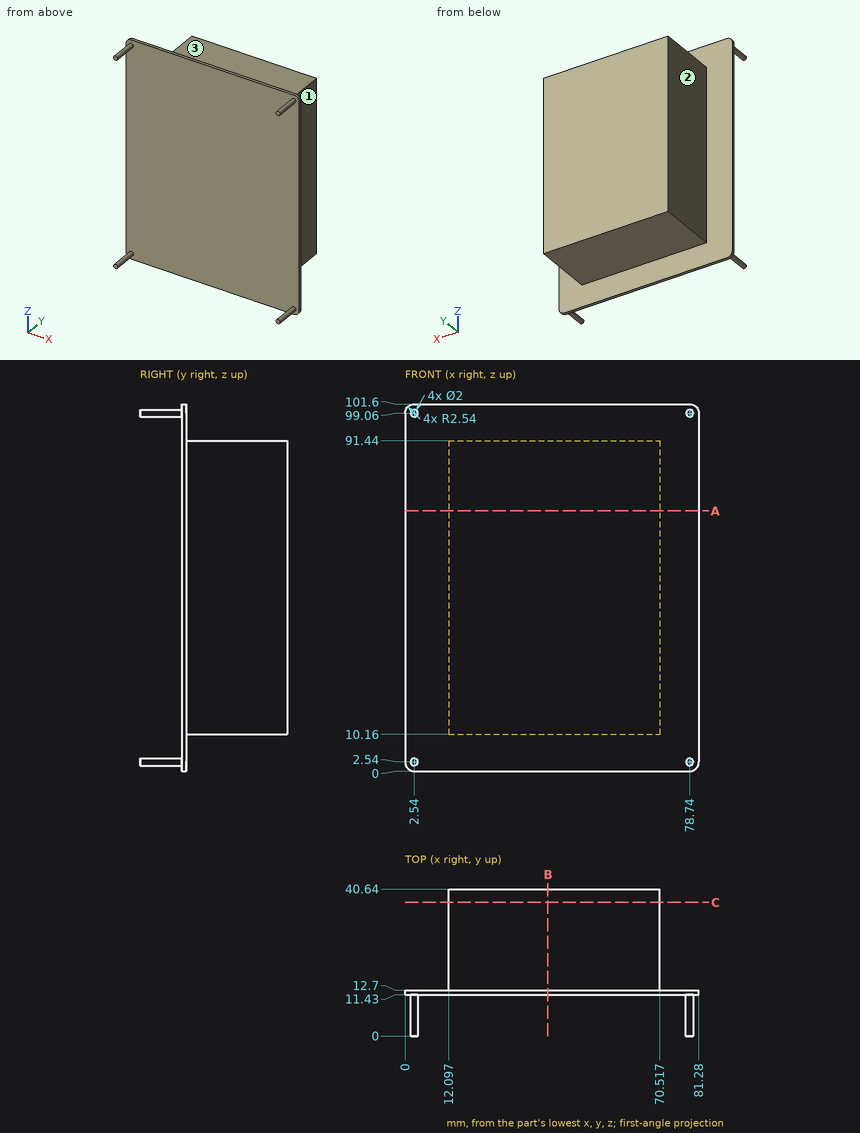
Verification items for this drawing (mm, ordinates from the low corner). A direction names the side the tool comes from. Give positions to 0.01 mm unless a question says otherwise; leave off trailing zeros. Write each loop counter-clockwise with the first axis right and the second up, starting at its lowest first coordinate (ties: lowest second). Pieces come first, ordered by that corner, then holes. Notation, with made-up numbers: (-1.5, -13) - (45.5, -13) arc R24 ccw to (45.5, -3) - close; hole circle Ø5 at (34, 33). An arc over 180 degrees is marked (long way). Answer as a JSON object with one key per item and string values. Group by question number.
1) Sectioned sample at C-C (y = 37). Record the cut outline in (x, z), then the cut area to 3 significant figures.
2) Depth check by flat-ended pin: P1, Ø2, axis at x = 13, z = 76.5, coming from the -Y side; P2, Ø14, axis at x = 35, y = 23, coming from the +Z side; P3, Ø22.5, axis at y = 26.5, z = 37.5, coming from the -X side. Enter the tip coordinate at first touch or a pass-through.
3) Sectioned sample at B-B (x = 39.5). Record the cut outline in (y, z).
4) Sectioned sample at A-A (z = 72). Record the cut outline in (x, y).
5) Access from +Z, -Z, +X, -X, +Y, -Y to the whole of each face (thin tool, end or side, straight path). Record for the marked faces 1, 2 and 3.
6) Thickness scan on probe 1 along Y at (x, z) = (78.5, 13); probe 2 along X at (y, z) = (30, 14); probe 3 along Z at (x, y) = (58, 25). Record the ranges inside material, lowest first. Write a range as from..to.
Geometry results:
{
 "1": {"outline": "(12.1, 10.16) - (70.52, 10.16) - (70.52, 91.44) - (12.1, 91.44) - close", "area": "4,750 mm^2"},
 "2": {"P1": "stops at y = 11.43", "P2": "stops at z = 91.44", "P3": "stops at x = 12.1"},
 "3": {"outline": "(11.43, 0) - (12.7, 0) - (12.7, 10.16) - (40.64, 10.16) - (40.64, 91.44) - (12.7, 91.44) - (12.7, 101.6) - (11.43, 101.6) - close"},
 "4": {"outline": "(0, 11.43) - (81.28, 11.43) - (81.28, 12.7) - (70.52, 12.7) - (70.52, 40.64) - (12.1, 40.64) - (12.1, 12.7) - (0, 12.7) - close"},
 "5": {"face 1": "+Z, -Z, +X, +Y", "face 2": "+Z, -Z, -X, +Y", "face 3": "+Z, +X, -X, +Y"},
 "6": {"probe 1": "y = 11.43..12.7", "probe 2": "x = 12.1..70.52", "probe 3": "z = 10.16..91.44"}
}
